from build123d import *

# Parameters (mm, degrees)
SKETCH_1_W      = 22.4
SKETCH_1_H      = 12.5
EXTRUDE_1_DEPTH = 16.1
SKETCH_2_W      = 31.8
SKETCH_2_H      = 12.5
EXTRUDE_2_DEPTH = 2
SKETCH_3_W      = 22.4
SKETCH_3_H      = 12.5
EXTRUDE_3_DEPTH = 4.7
SKETCH_4_R      = 6.25
EXTRUDE_4_DEPTH = 9.3


with BuildPart() as part:
    # 草图1 → 凸台-拉伸1 (new body)
    with BuildSketch(Plane.XY):
        Rectangle(SKETCH_1_W, SKETCH_1_H)
    extrude(amount=EXTRUDE_1_DEPTH)

    # 草图2 → 凸台-拉伸2 (add)
    with BuildSketch(Plane(origin=(0, 0, 0), x_dir=(-1, 0, 0), z_dir=(0, 0, -1))):
        Rectangle(SKETCH_2_W, SKETCH_2_H)
    extrude(amount=EXTRUDE_2_DEPTH)

    # 草图3 → 凸台-拉伸3 (add)
    with BuildSketch(Plane(origin=(0, 0, -2), x_dir=(-1, 0, 0), z_dir=(0, 0, -1))):
        Rectangle(SKETCH_3_W, SKETCH_3_H)
    extrude(amount=EXTRUDE_3_DEPTH)

    # 草图4 → 凸台-拉伸4 (add)
    with BuildSketch(Plane(origin=(0, 0, -6.7), x_dir=(-1, 0, 0), z_dir=(0, 0, -1))):
        with Locations(Location((-4.95, 0, 0), (0, 0, 180))):
            Circle(SKETCH_4_R)
    extrude(amount=EXTRUDE_4_DEPTH)


solid = part.part
Input: part model. Units: mm. Frame: model coordinates. A direction names the side the tool comes from. Round coordinates to 2 decimals unless told otherwise and drop trailing zeros. Order: outer loops, then holes, each group sorted by start corner. A loop starts at its lowest first (then second) coordinate and runs counter-clockwise, first axis right, second up. Notation, with made-up numbers: (-10.75, -16) - (18.25, -16) arc R17 cw to (18.25, -6) - close; hole circle Ø3 at (23, 45). An arc over 180 degrees is marked (long way). Use a Markdown table: item, result.
1. Section B-B on z = 14.5. Return the cut outline in (x, y).
Evaluation:
| item | result |
|---|---|
| outline | (-11.2, -6.25) - (11.2, -6.25) - (11.2, 6.25) - (-11.2, 6.25) - close |
2. Access query for faces 1 (the face through (-14, 0, 0)), 2 (the face through (11.2, 0, 8)), 3 (the face through (10, -5, -6.7)), 4 (the face through (10, 5, -6.7)). Directions: +Z, -Z, +X, -X, +Y, -Y. A direction counts if a zero-diameter tool reaches every point of the face in a straight line with its end or side. Return the directions, or none.
Evaluation:
| item | result |
|---|---|
| face 1 | +Z, -X, +Y, -Y |
| face 2 | +Z, +X, +Y, -Y |
| face 3 | -Z, +X, -Y |
| face 4 | -Z, +X, +Y |
3. Material intervals for probe 1 along X at (y, z) = (-4.25, 14.5); probe 2 along Z at (x, y) = (1.5, -5.25); probe 3 along Z at (x, y) = (-13, -3.75), sorted ascending.
Evaluation:
| item | result |
|---|---|
| probe 1 | -11.2 to 11.2 |
| probe 2 | -6.7 to 16.1 |
| probe 3 | -2 to 0 |
4. Section C-C on x = -6.5. Return the cut outline in (y, z), then the cut area to 3 significant figures.
Evaluation:
| item | result |
|---|---|
| outline | (-6.25, -6.7) - (6.25, -6.7) - (6.25, 16.1) - (-6.25, 16.1) - close |
| area | 285 mm^2 |
5. First-contact query: pin 1 (4 mm diameter, centred on y = 0, z = 4.5, fed in from -X); pin 2 (1.4 mm diameter, centred on x = 13, y = -1, fed in from -Z); pin 3 (1.5 mm diameter, centred on x = -10.5, y = 4, fed in from -Z). Flat tips, straight axial feed; report the tip coordinate or a pass-through.
Evaluation:
| item | result |
|---|---|
| pin 1 | x = -11.2 |
| pin 2 | z = -2 |
| pin 3 | z = -6.7 |
6. Section A-A on y = -3.25. Return the cut outline in (x, z).
Evaluation:
| item | result |
|---|---|
| outline | (-15.9, -2) - (-11.2, -2) - (-11.2, -6.7) - (-0.39, -6.7) - (-0.39, -16) - (10.29, -16) - (10.29, -6.7) - (11.2, -6.7) - (11.2, -2) - (15.9, -2) - (15.9, 0) - (11.2, 0) - (11.2, 16.1) - (-11.2, 16.1) - (-11.2, 0) - (-15.9, 0) - close |
